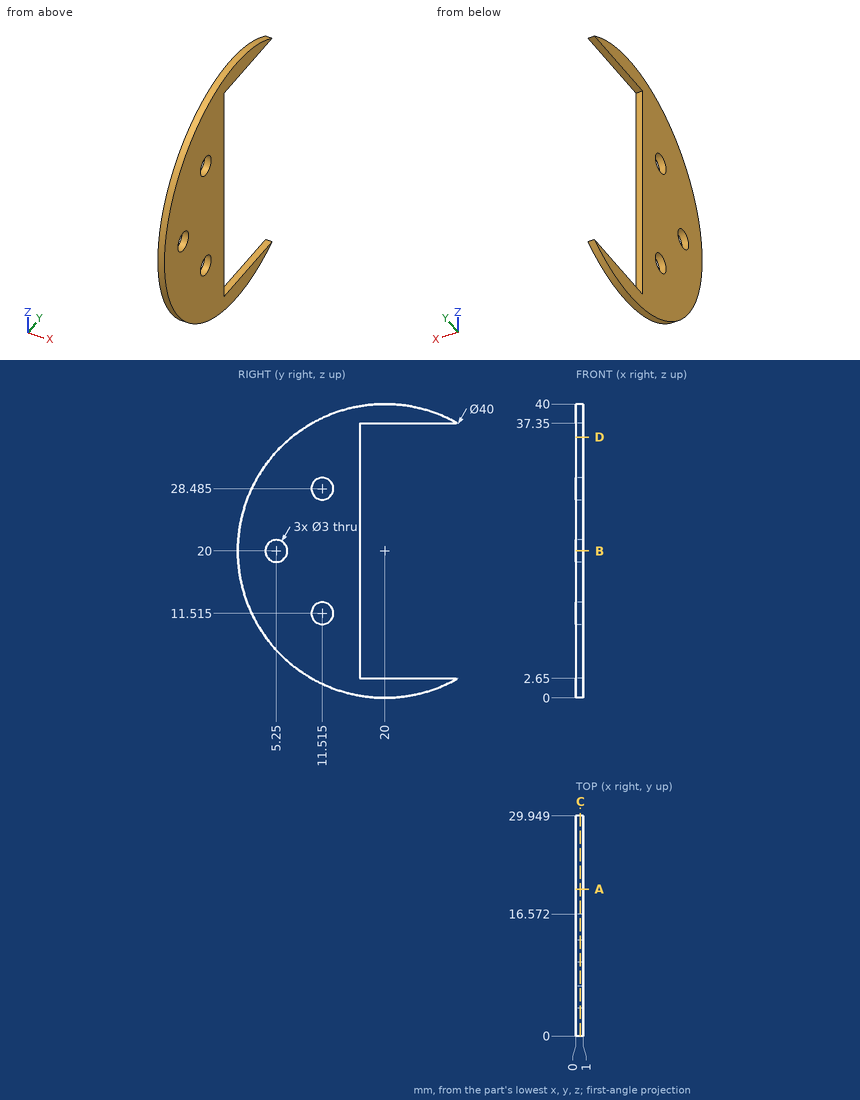
The figure shows three views and two pictorial views of one solid part (mm, origin at its lowest corner). Answer the questions. Coordinates: 2 decimals unless noted, no trailing zeros. Write each loop counter-clockwise with the first axis right and the second up, starting at its lowest first coordinate (ties: lowest second). Pieces come first, ordered by that corner, then holes.
1. The part is cut by section C-C, the plane x = 0.6. State how many separate pieces and enclosed holes the cut face has, and give its area (3 significant figures).
Results list:
separate pieces: 1
enclosed holes: 3
area: 524 mm2
2. Consider line 1 along Y through (x, z) = (0.75, 20); line 2 along Z through (x, y) = (0.55, 17); line 3 along Z through (x, y) = (0.55, 21.5). Determine where each line is inside the solid, lowest interval first.
Results list:
line 1: y = 0 to 3.75, 6.75 to 16.57
line 2: z = 0.23 to 2.65, 37.35 to 39.77
line 3: z = 0.06 to 2.65, 37.35 to 39.94
3. The part is cut by section D-D, the plane z = 35.5. Write down the section's boundary in (x, y).
Results list:
outline: (0, 7.36) - (1, 7.36) - (1, 16.57) - (0, 16.57) - close
4. The part is cut by section B-B, the plane z = 20. Write down the section's boundary in (x, y).
Results list:
outline: (0, 0) - (1, 0) - (1, 3.75) - (0, 3.75) - close; (0, 6.75) - (1, 6.75) - (1, 16.57) - (0, 16.57) - close
5. The part is cut by section A-A, the plane y = 20. Write down the section's boundary in (x, z).
Results list:
outline: (0, 0) - (1, 0) - (1, 2.65) - (0, 2.65) - close; (0, 37.35) - (1, 37.35) - (1, 40) - (0, 40) - close
